Geometry check sheet. Reference: the model listing, model coordinates, mm. Coordinates: 2 decimals unless noted, no trailing zeros. Write each loop counter-clockwise with the first axis right and the second up, starting at its lowest first coordinate (ties: lowest second). Pieces come first, ordered by that corner, then holes. Notation, with made-up numbers: (-12, 45) -> (27, 45) arc R15 cw to (27, 55) -> close; hole circle Ø8 at (58.25, -8.5). An arc over 180 degrees is marked (long way). Answer in a Markdown table with one row per item. Add a question column.
Q1. Section check A-A, the plane y = 133. Record the boundary of the cut face in (x, z), and give its area (3 significant figures).
Q2. Section check B-B, the plane z = 4.45. Count the separate pieces of the cut face and the enclosed holes in it, and give its area (3 significant figures).
Q3. Thickness scan on line 1 (Y direction, x = 20.5, z = 5.3); line 2 (X direction, y = 20.5, z = 3.4); line 3 (Y direction, x = 39, z = 3). Record the ranges inside material, lowest first.
Q4. Release check for a two-part mould opening along X. For faces 1 (the face through (-5, 27, 0)), 2 (the face through (2.8, 38, 3)) record: pulls with the +X half, pulls with the -X half, needs draft (parallel to the pull), parting line crosses it, or undercut.
```python
from build123d import *

# Parameters (mm, degrees)
SKETCH1_R           = 1.5
SKETCH1_R_2         = 22.511799613
BOSS_EXTRUDE1_DEPTH = 6


with BuildPart() as part:
    # Sketch1 → Boss-Extrude1 (new body)
    with BuildSketch(Plane.XY):
        Polygon((114.346400169, -107.26425955), (114.346400169, -67.26425955), (120.346400169, -67.26425955), (120.346400169, -7.26425955), (114.346400169, -7.26425955), (114.346400169, 52.73574045), (120.346400169, 52.73574045), (120.346400169, 112.73574045), (114.346400169, 112.73574045), (114.346400169, 152.73574045), (120.346400169, 152.73574045), (120.346400169, 212.73574045), (114.346400169, 212.73574045), (114.346400169, 262.73574045), (120.346400169, 262.73574045), (120.346400169, 317.807433635), (-81.653599831, 317.807433635), (-81.653599831, 262.73574045), (-75.653599831, 262.73574045), (-75.653599831, 212.73574045), (-81.653599831, 212.73574045), (-81.653599831, 152.73574045), (-75.653599831, 152.73574045), (-75.653599831, 112.73574045), (-81.653599831, 112.73574045), (-81.653599831, 52.73574045), (-75.653599831, 52.73574045), (-75.653599831, -7.26425955), (-81.653599831, -7.26425955), (-81.653599831, -67.26425955), (-75.653599831, -67.26425955), (-75.653599831, -107.26425955), (-81.653599831, -107.26425955), (-81.653599831, -167.26425955), (-75.653599831, -167.26425955), (-75.653599831, -217.26425955), (-81.653599831, -217.26425955), (-81.653599831, -272.335952735), (120.346400169, -272.335952735), (120.346400169, -217.26425955), (114.346400169, -217.26425955), (114.346400169, -167.26425955), (120.346400169, -167.26425955), (120.346400169, -107.26425955), align=None)
        with Locations((93.421400169, 144.187215683)):
            Circle(SKETCH1_R, mode=Mode.SUBTRACT)
        with Locations((93.421400169, 176.66641252)):
            Circle(SKETCH1_R, mode=Mode.SUBTRACT)
        with Locations((33.421400169, 144.187215683)):
            Circle(SKETCH1_R, mode=Mode.SUBTRACT)
        with Locations((-54.728599831, -131.19493162)):
            Circle(SKETCH1_R, mode=Mode.SUBTRACT)
        with Locations((33.421400169, 176.66641252)):
            Circle(SKETCH1_R, mode=Mode.SUBTRACT)
        with Locations((-54.728599831, -98.715734783)):
            Circle(SKETCH1_R, mode=Mode.SUBTRACT)
        with Locations((5.271400169, -98.715734783)):
            Circle(SKETCH1_R, mode=Mode.SUBTRACT)
        with Locations((19.346400169, 22.73574045)):
            Circle(SKETCH1_R_2, mode=Mode.SUBTRACT)
        with Locations((5.271400169, -131.19493162)):
            Circle(SKETCH1_R, mode=Mode.SUBTRACT)
        with BuildLine():
            Line((41.149833216, -2.603226503), (37.611612305, 0.934994409))
            ThreePointArc((37.611612305, 0.934994409), (37.611612305, 4.470528314), (41.147146211, 4.470528314))
            Line((41.147146211, 4.470528314), (44.685367122, 0.932307403))
            ThreePointArc((44.685367122, 0.932307403), (44.685367122, -2.603226503), (41.149833216, -2.603226503))
        make_face(mode=Mode.SUBTRACT)
        with BuildLine():
            Line((-5.992566784, 0.932307403), (-2.454345872, 4.470528314))
            ThreePointArc((-2.454345872, 4.470528314), (1.081188034, 4.470528314), (1.081188034, 0.934994409))
            Line((1.081188034, 0.934994409), (-2.457032878, -2.603226503))
            ThreePointArc((-2.457032878, -2.603226503), (-5.992566784, -2.603226503), (-5.992566784, 0.932307403))
        make_face(mode=Mode.SUBTRACT)
        with BuildLine():
            Line((-2.457032878, 48.074707403), (1.081188034, 44.536486491))
            ThreePointArc((1.081188034, 44.536486491), (1.081188034, 41.000952585), (-2.454345872, 41.000952585))
            Line((-2.454345872, 41.000952585), (-5.992566784, 44.539173497))
            ThreePointArc((-5.992566784, 44.539173497), (-5.992566784, 48.074707403), (-2.457032878, 48.074707403))
        make_face(mode=Mode.SUBTRACT)
        with BuildLine():
            Line((44.685367122, 44.539173497), (41.147146211, 41.000952585))
            ThreePointArc((41.147146211, 41.000952585), (37.611612305, 41.000952585), (37.611612305, 44.536486491))
            Line((37.611612305, 44.536486491), (41.149833216, 48.074707403))
            ThreePointArc((41.149833216, 48.074707403), (44.685367122, 48.074707403), (44.685367122, 44.539173497))
        make_face(mode=Mode.SUBTRACT)
    extrude(amount=BOSS_EXTRUDE1_DEPTH)


solid = part.part
```
Calculated:
| question | item | result |
|---|---|---|
| 1 | outline | (-75.65, 0) -> (114.35, 0) -> (114.35, 6) -> (-75.65, 6) -> close |
| 1 | area | 1,140 mm² |
| 2 | separate pieces | 1 |
| 2 | enclosed holes | 13 |
| 2 | area | 115,000 mm² |
| 3 | line 1 | y = -272.34 to 0.25, 45.22 to 317.81 |
| 3 | line 2 | x = -75.65 to -3.05, 41.75 to 114.35 |
| 3 | line 3 | y = -272.34 to -0.45, 5.17 to 11.76, 33.71 to 40.3, 45.92 to 317.81 |
| 4 | face 1 | needs draft |
| 4 | face 2 | undercut |
